Could you check a few things on this model? Use its own coordinates, in mm. A direction names the side the tool comes from. Coordinates: 2 decimals unless noted, no trailing zeros. Order: outer loops, then holes, each group sorted by start corner. A loop starts at its lowest first (then second) coordinate and runs counter-clockwise, first axis right, second up. Notation, with made-up numbers: (6.5, 13.5) -> (27.5, 13.5) arc R22 cw to (27.5, 23.5) -> close; hole circle Ø9 at (-5, 40.25). An arc over 180 degrees is marked (long way). Use a Markdown table: item, result. Add a question column.
1) If we section it at D-D (z = -13.5): Write out the boundary of the cut face in (x, y).
2) Which directions (+Z, -Z, +X, -X, +Y, -Y) give clear straight access to the entire face, cutting with the end or side of a thin tool? Please do faces 1 (the flat face through (5, -1.054, -16)), 2 (the cylindrical face through (-6.43, 19.5, -26.79)), 3 (the flat face through (-44, 16.946, -1)), 4 (the cylindrical face through (-45.451, -0.626, -16.143)), 5 (the cylindrical face through (-50.119, -2.575, -33.435)).
3) Will these pins go through, and if not, where does the flat tip stop? pin 1 Ø0.9 at (x, z) = (-4, -6) entering from +Y; pin 2 Ø8 at (x, z) = (-24, -18.76) entering from -Y; pin 3 Ø1 at (y, z) = (5, -34) entering from +X; pin 4 Ø5.5 at (x, z) = (-24, -30.76) entering from -Y.
4) If we section it at C-C (y = 10.25): Write out the boundary of the cut face in (x, z).
5) If we section it at A-A (z = -6.5): Write out the boundary of the cut face in (x, y), plus the area to 3 significant figures.
6) If I drill on L1, parallel to Z at x = -52.5, y = -2.5; L2, parallel to X at y = 1.5, z = -35.5; L3, parallel to Z at x = -24, y = 21.15, over which ranges is the centre line in solid material (lowest first)? Write a range as [from, to].
7) If we section it at B-B (x = -24): Write out the boundary of the cut face in (y, z), plus the area to 3 significant figures.
8) Thinking about a two-plate mould opening in Z: for faces 6 (the flat face through (-45, 9, -16)), 7 (the cylindrical face through (5.15, -2.575, -32.332)), 8 (the flat face through (-24, 21, -11.261)), which applies, +Z half, -Z half, draft (parallel to the pull), parting line (faces both ways), or undercut?
```python
from build123d import *

# Parameters (mm, degrees)
BASE_FLANGE1_DEPTH                 = 35
SKETCH10_W                         = 28
SKETCH10_H                         = 14
CUT_EXTRUDE1_DEPTH                 = 4
F_4_0_4_DIAMETER_HOLE1_D           = 4
F_4_0_4_DIAMETER_HOLE1_CSINK_D     = 4.05
F_4_0_4_DIAMETER_HOLE1_CSINK_ANGLE = 90
SCALE1_SCALE                       = 1.5


# Sheet-metal steps are written as plain solids
with BuildPart() as part:
    # Sketch1 → Base-Flange1 (new body)
    with BuildSketch(Plane.XY):
        with BuildLine():
            Line((0, 0), (-9, 0))
            ThreePointArc((-9, 0), (-11.121320344, 0.878679656), (-12, 3))
            Line((-12, 3), (-12, 15))
            ThreePointArc((-12, 15), (-12.292893219, 15.707106781), (-13, 16))
            Line((-13, 16), (-35, 16))
            ThreePointArc((-35, 16), (-35.707106781, 15.707106781), (-36, 15))
            Line((-36, 15), (-36, 3))
            ThreePointArc((-36, 3), (-36.878679656, 0.878679656), (-39, 0))
            Line((-39, 0), (-48, 0))
            Line((-48, 0), (-48, 2))
            Line((-48, 2), (-39, 2))
            ThreePointArc((-39, 2), (-38.292893219, 2.292893219), (-38, 3))
            Line((-38, 3), (-38, 15))
            ThreePointArc((-38, 15), (-37.121320344, 17.121320344), (-35, 18))
            Line((-35, 18), (-13, 18))
            ThreePointArc((-13, 18), (-10.878679656, 17.121320344), (-10, 15))
            Line((-10, 15), (-10, 3))
            ThreePointArc((-10, 3), (-9.707106781, 2.292893219), (-9, 2))
            Line((-9, 2), (0, 2))
            Line((0, 2), (0, 0))
        make_face()
    extrude(amount=-BASE_FLANGE1_DEPTH)

    # Sketch10 → Cut-Extrude1 (cut)
    with BuildSketch(Plane(origin=(0, 18, 0), x_dir=(1, 0, 0), z_dir=(0, 1, 0))):
        with Locations((-24, 7)):
            Rectangle(SKETCH10_W, SKETCH10_H)
    extrude(amount=-CUT_EXTRUDE1_DEPTH, mode=Mode.SUBTRACT)

    # Ø4.0 (4) Diameter Hole1 (through all)
    with Locations(Plane(origin=(0, 18, 0), x_dir=(1, 0, 0), z_dir=(0, 1, 0))):
        with Locations((-24, 27), (-24, 19), (-43, 30), (-43, 5), (-5, 30), (-5, 5)):
            CounterSinkHole(F_4_0_4_DIAMETER_HOLE1_D / 2, F_4_0_4_DIAMETER_HOLE1_CSINK_D / 2, counter_sink_angle=F_4_0_4_DIAMETER_HOLE1_CSINK_ANGLE)


with BuildPart() as part_1:
    # Scale1: scaled about (-24, 8.107482912, -19.478199083)
    add(part.part.scale(SCALE1_SCALE).moved(Location((12, -4.053741456, 9.739099541))))


solid = part_1.part
```
Answer sheet:
| question | item | result |
|---|---|---|
| 1 | outline | (-60, -4.05) -> (-46.5, -4.05) arc R4.5 ccw to (-42, 0.45) -> (-42, 18.45) arc R1.5 cw to (-40.5, 19.95) -> (-7.5, 19.95) arc R1.5 cw to (-6, 18.45) -> (-6, 0.45) arc R4.5 ccw to (-1.5, -4.05) -> (12, -4.05) -> (12, -1.05) -> (-1.5, -1.05) arc R1.5 cw to (-3, 0.45) -> (-3, 18.45) arc R4.5 ccw to (-7.5, 22.95) -> (-40.5, 22.95) arc R4.5 ccw to (-45, 18.45) -> (-45, 0.45) arc R1.5 cw to (-46.5, -1.05) -> (-60, -1.05) -> close |
| 2 | face 1 | +Z, -Z, +X, +Y |
| 2 | face 2 | +Z, -Z, -Y |
| 2 | face 3 | +Z, +X, -X, +Y |
| 2 | face 4 | +Z, -Z, -X, +Y |
| 2 | face 5 | +Y, -Y |
| 3 | pin 1 | y = 16.95 |
| 3 | pin 2 | y = 19.95 |
| 3 | pin 3 | x = -3 |
| 3 | pin 4 | through |
| 4 | outline | (-45, -42.76) -> (-42, -42.76) -> (-42, 9.74) -> (-45, 9.74) -> close; (-6, -42.76) -> (-3, -42.76) -> (-3, 9.74) -> (-6, 9.74) -> close |
| 5 | outline | (-60, -4.05) -> (-46.5, -4.05) arc R4.5 ccw to (-42, 0.45) -> (-42, 16.95) -> (-45, 16.95) -> (-45, 0.45) arc R1.5 cw to (-46.5, -1.05) -> (-60, -1.05) -> close; (-6, 0.45) arc R4.5 ccw to (-1.5, -4.05) -> (12, -4.05) -> (12, -1.05) -> (-1.5, -1.05) arc R1.5 cw to (-3, 0.45) -> (-3, 16.95) -> (-6, 16.95) -> close |
| 5 | area | 208 mm2 |
| 6 | L1 | [-42.76, -38.26], [-32.26, -0.76], [5.24, 9.74] |
| 6 | L2 | [-45, -42], [-6, -3] |
| 6 | L3 | [-42.76, -33.76], [-27.76, -21.76], [-15.76, -11.26] |
| 7 | outline | (19.95, -42.76) -> (22.95, -42.76) -> (22.95, -33.8) -> (22.91, -33.76) -> (19.95, -33.76) -> close; (19.95, -27.76) -> (22.91, -27.76) -> (22.95, -27.72) -> (22.95, -21.8) -> (22.91, -21.76) -> (19.95, -21.76) -> close; (19.95, -15.76) -> (22.91, -15.76) -> (22.95, -15.72) -> (22.95, -11.26) -> (19.95, -11.26) -> close |
| 7 | area | 58.5 mm2 |
| 8 | face 6 | draft |
| 8 | face 7 | undercut |
| 8 | face 8 | +Z half |
